Autodesk Inventor part; units mm, degrees
ref_plane "YZ Plane" through (0, 0, 0) normal (1, 0, 0) x (0, 1, 0)
ref_plane "XZ Plane" through (0, 0, 0) normal (0, 1, 0) x (-1, 0, 0)
ref_plane "XY Plane" through (0, 0, 0) normal (0, 0, 1) x (1, 0, 0)
sketch "Sketch1" plane through (0, 0, 0) normal (0, 0, 1) x (1, 0, 0)
  line L0 (0, 0) -> (25.4, 0)
  line L1 (25.4, 0) -> (25.4, 25.4)
  line L2 (25.4, 25.4) -> (0, 25.4)
  line L3 (0, 25.4) -> (0, 0)
  dimension "d0" = 25.4
  dimension "d1" = 25.4
extrude "Extrusion1" add sketch "Sketch1" along normal blind 609.6
shell "Shell1" thickness 2.54 removed faces 2 at (8.4667, 16.9333, 0) at (8.4667, 16.9333, 609.6)
sketch "Sketch2" plane through (0, 25.4, 0) normal (0, 1, 0) x (1, 0, 0)
  line L0 (25.4, 0) -> (0, 0)
  line L1 (0, 0) -> (0, -609.6)
  point P0 (12.7, -12.7)
  point P1 (12.7, -38.1)
  point P2 (12.7, -63.5)
  point P3 (12.7, -88.9)
  point P4 (12.7, -114.3)
  point P5 (12.7, -139.7)
  point P6 (12.7, -165.1)
  point P7 (12.7, -190.5)
  point P8 (12.7, -215.9)
  point P9 (12.7, -241.3)
  point P10 (12.7, -266.7)
  point P11 (12.7, -292.1)
  point P12 (12.7, -317.5)
  point P13 (12.7, -342.9)
  point P14 (12.7, -368.3)
  point P15 (12.7, -393.7)
  point P16 (12.7, -419.1)
  point P17 (12.7, -444.5)
  point P18 (12.7, -469.9)
  point P19 (12.7, -495.3)
  point P20 (12.7, -520.7)
  point P21 (12.7, -546.1)
  point P22 (12.7, -571.5)
  point P23 (12.7, -596.9)
  point P24 (12.7, -622.3)
  point P25 (12.7, -647.7)
  point P26 (12.7, -673.1)
  point P27 (12.7, -698.5)
  point P28 (12.7, -723.9)
  point P29 (12.7, -749.3)
  point P30 (12.7, -774.7)
  point P31 (12.7, -800.1)
  point P32 (12.7, -825.5)
  point P33 (12.7, -850.9)
  point P34 (12.7, -876.3)
  point P35 (12.7, -901.7)
  point P36 (12.7, -927.1)
  dimension "d5" = 12.7
  dimension "d6" = 12.7
  dimension "d9" = 25.4
hole "Hole1" at (12.7, 25.4, 12.7) at (12.7, 25.4, 38.1) at (12.7, 25.4, 63.5) at (12.7, 25.4, 88.9) at (12.7, 25.4, 114.3) at (12.7, 25.4, 139.7) at (12.7, 25.4, 165.1) at (12.7, 25.4, 190.5) at (12.7, 25.4, 215.9) at (12.7, 25.4, 241.3) at (12.7, 25.4, 266.7) at (12.7, 25.4, 292.1) at (12.7, 25.4, 317.5) at (12.7, 25.4, 342.9) at (12.7, 25.4, 368.3) at (12.7, 25.4, 393.7) at (12.7, 25.4, 419.1) at (12.7, 25.4, 444.5) at (12.7, 25.4, 469.9) at (12.7, 25.4, 495.3) at (12.7, 25.4, 520.7) at (12.7, 25.4, 546.1) at (12.7, 25.4, 571.5) at (12.7, 25.4, 596.9) at (12.7, 25.4, 622.3) at (12.7, 25.4, 647.7) at (12.7, 25.4, 673.1) at (12.7, 25.4, 698.5) at (12.7, 25.4, 723.9) at (12.7, 25.4, 749.3) at (12.7, 25.4, 774.7) at (12.7, 25.4, 800.1) at (12.7, 25.4, 825.5) at (12.7, 25.4, 850.9) at (12.7, 25.4, 876.3) at (12.7, 25.4, 901.7) direction (0, -1, 0) diameter 2.54 depth 50.8 tip angle 118
properties part number "Electric Board Upright" material "Aluminum 6061"
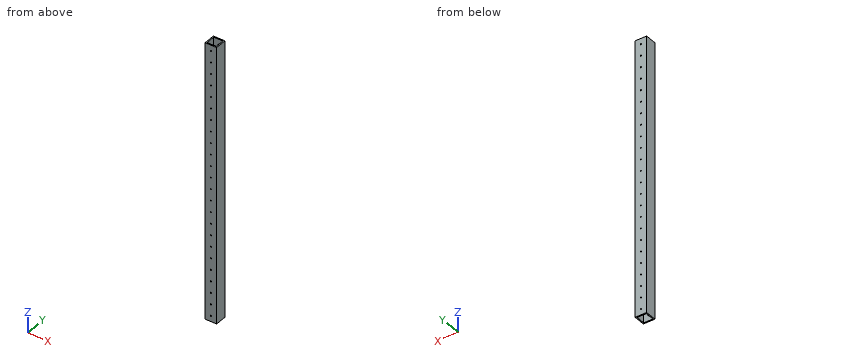
For this review, take the finished solid that the model builds, in its own axes (mm). Coordinates: 2 decimals unless noted, no trailing zeros. Order: outer loops, then holes, each group sorted by start corner. A loop starts at its lowest first (then second) coordinate and runs counter-clockwise, first axis right, second up. Notation, with made-up numbers: (-25, 66) - (5, 66) arc R15 ccw to (5, 93) - close; hole circle Ø4 at (-21, 50). An arc over 180 degrees is marked (long way). Answer as a JSON object with one key per item and string values. Group by question number.
1. We need section B-B on z = 284.5. State the section outline as (x, y) points, then the cut area to 3 significant figures.
2. For probe 1 along Y at (x, z) = (11.25, 511); probe 2 along X at (y, z) = (1.3, 114.3), list the stretches that pass through material, from the lowest coordinate up.
3. We need section A-A on y = 12.5. State the section outline as (x, z) points, then the cut area to 3 significant figures.
4. Clearance check with a flat-ended pin moving along its axis: P1, Ø1.5, axis at x = 12.7, z = 342.9, coming from the -Y side. State where the tip first meets the part, or that it passes through.
Final values:
{
 "1": {"outline": "(0, 0) - (25.4, 0) - (25.4, 25.4) - (0, 25.4) - close; hole (2.54, 2.54) - (22.86, 2.54) - (22.86, 22.86) - (2.54, 22.86) - close", "area": "232 mm²"},
 "2": {"probe 1": "0 to 2.54, 22.86 to 25.4", "probe 2": "0 to 11.43, 13.97 to 25.4"},
 "3": {"outline": "(0, 0) - (2.54, 0) - (2.54, 609.6) - (0, 609.6) - close; (22.86, 0) - (25.4, 0) - (25.4, 609.6) - (22.86, 609.6) - close", "area": "3,100 mm²"},
 "4": {"P1": "through"}
}
